Read the model definition and answer for the solid it produces. Units are mm, in the model's axes. A direction names the side the tool comes from. Give positions to 0.01 mm unless a question says otherwise; leave off trailing zeros. Write each loop counter-clockwise with the first axis right and the second up, starting at its lowest first coordinate (ties: lowest second). Pieces come first, ordered by that corner, then holes.
```python
from build123d import *

# Parameters (mm, degrees)
F1_DEPTH = 12.7
F2_R     = 3.302
F3_DEPTH = 25.4


with BuildPart() as f1:
    # F0 (on Top) → F1 (new body)
    with BuildSketch(Plane.XY):
        with BuildLine():
            ThreePointArc((25.232093, 2.915727), (16.898233, 18.963379), (0, 25.4))
            ThreePointArc((0, 25.4), (-17.960512, -17.960512), (25.4, 0))
            ThreePointArc((25.4, 0), (25.331587, 1.458758), (25.232093, 2.915727))
        make_face()
        with BuildLine():
            Line((0, 50.8), (0, 25.4))
            ThreePointArc((0, 25.4), (16.898233, 18.963379), (25.232093, 2.915727))
            ThreePointArc((25.232093, 2.915727), (17.545737, 29.455509), (0, 50.8))
        make_face()
    extrude(amount=F1_DEPTH)

    # F2 (on face) → F3 (cut)
    with BuildSketch(Plane.XY.offset(12.7)):
        Circle(F2_R)
    extrude(amount=-F3_DEPTH, mode=Mode.SUBTRACT)


solid = f1.part
```
Item 1: Section A-A (z = 2.5) is taken. Write down the section's boundary in (x, y), and give its area (3 significant figures).
Result set:
outline: (0, 25.4) arc R25.4 ccw (long way) to (25.4, 0) arc R68.5 ccw to (25.23, 2.92) arc R68.5 ccw to (0, 50.8) - close; hole circle Ø6.6 at (0, 0)
area: 2,370 mm2
Item 2: Determine the mould class of faces 3 (the cylindrical face through (3.05, -1.26, 6.44)), 4 (the flat face through (0, 5, 0)), 5 (the cylindrical face through (25.333, 1.438, 6.261)) for opening direction Y: pulls with the +Y half, pulls with the -Y half, needs draft (parallel to the pull), parting line crosses it, or undercut.
Result set:
face 3: undercut
face 4: needs draft
face 5: pulls with the +Y half
Item 3: Which of the six approach directions +Z, -Z, +X, -X, +Y, -Y give full straight-line access (tool end or side, diameter ignored) to faces 1 (the flat face through (0, 38, 6)), 2 (the cylindrical face through (17.726, 29.11, 6.261))?
Result set:
face 1: +Z, -Z, -X, +Y
face 2: +Z, -Z, +X, +Y
Item 4: Section B-B (y = 5) is taken. Write down the section's boundary in (x, z), and give its area (3 significant figures).
Result set:
outline: (-24.9, 0) - (25.04, 0) - (25.04, 12.7) - (-24.9, 12.7) - close
area: 634 mm2
Item 5: Section C-C (x = 10) is taken. Write down the section's boundary in (y, z), and give its area (3 significant figures).
Result set:
outline: (-23.35, 0) - (40.85, 0) - (40.85, 12.7) - (-23.35, 12.7) - close
area: 815 mm2
Item 6: Each of these flat-tipped pins is pushed along its axis until it touches: pin 1 Ø1.5 at (x, z) = (-9.5, 2.5) entering from -Y; pin 2 Ø1 at (y, z) = (-14.5, 3) entering from -X; pin 3 Ø2 at (x, z) = (19.5, 9) entering from +Y. Where does it stop, or does it pass through?
Result set:
pin 1: stops at y = -23.85
pin 2: stops at x = -21.19
pin 3: stops at y = 27.57
Item 7: Find the intervals of material crossed by line 1 along Y through (x, z) = (-17, 5.25); line 2 along Y through (x, z) = (-9, 3.25); line 3 along X through (y, z) = (28.5, 0.5), in increasing order.
Result set:
line 1: y = -18.87 to 18.87
line 2: y = -23.75 to 23.75
line 3: x = 0 to 18.04
